```python
from build123d import *

# Parameters (mm, degrees)
SKETCH1_W           = 36.576
SKETCH1_H           = 33.274
BOSS_EXTRUDE1_DEPTH = 1.499997
SKETCH2_W           = 19.05
SKETCH2_H           = 1.5875
SKETCH2_W_2         = 12.7
SKETCH2_W_3         = 9.525
SKETCH2_W_4         = 6.35
SKETCH2_W_5         = 15.875
BOSS_EXTRUDE2_DEPTH = 0.254


with BuildPart() as part:
    # Sketch1 → Boss-Extrude1 (new body)
    with BuildSketch(Plane(origin=(0, 0, 0), x_dir=(1, 0, 0), z_dir=(0, 1, 0))):
        Rectangle(SKETCH1_W, SKETCH1_H)
    extrude(amount=BOSS_EXTRUDE1_DEPTH)

    # Sketch2 → Boss-Extrude2 (add)
    with BuildSketch(Plane(origin=(0, 1.499997, 0), x_dir=(1, 0, 0), z_dir=(0, 1, 0))):
        with Locations((0, 0.66675)):
            Rectangle(SKETCH2_W, SKETCH2_H)
        with Locations((0, -6.31825)):
            Rectangle(SKETCH2_W_2, SKETCH2_H)
        with Locations((0, -9.81075)):
            Rectangle(SKETCH2_W_3, SKETCH2_H)
        with Locations((0, -13.30325)):
            Rectangle(SKETCH2_W_4, SKETCH2_H)
        with Locations((0, -2.82575)):
            Rectangle(SKETCH2_W_5, SKETCH2_H)
    extrude(amount=BOSS_EXTRUDE2_DEPTH)


solid = part.part
```
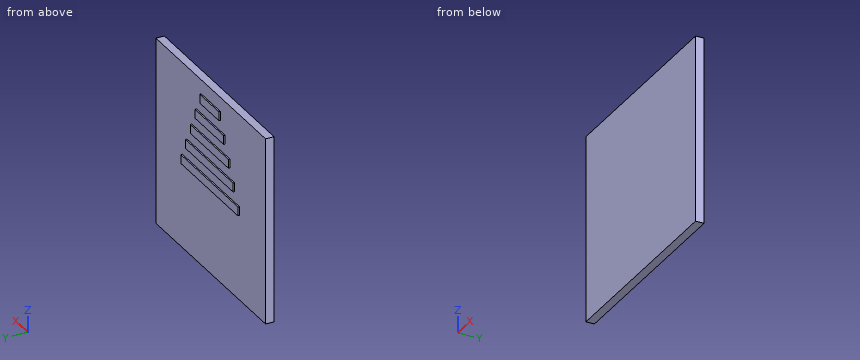
Verification items for the finished model (mm, model axes). Round coordinates to 2 decimals unless told otherwise and drop trailing zeros. Loops run counter-clockwise (first coordinate to the right, second up) from the corner with the lowest first, then second, coordinate; pieces in that order, holes last. Notation, with made-up numbers: (48, 28) -> (55, 28) arc R34 ccw to (55, 58) -> close; hole circle Ø8 at (11.25, 74). An arc over 180 degrees is marked (long way). Answer as a JSON object with one key per item and string values.
Q1. Section check D-D (z = 11.5). Record the boundary of the cut face in (x, y), then the cut area to 3 significant figures.
Data:
{"outline": "(-18.29, 0) -> (18.29, 0) -> (18.29, 1.5) -> (-18.29, 1.5) -> close", "area": "54.9 mm2"}
Q2. Section check A-A (x = -4). Record the boundary of the cut face in (y, z), then the cut area to 3 significant figures.
Data:
{"outline": "(0, -16.64) -> (1.5, -16.64) -> (1.5, -1.46) -> (1.75, -1.46) -> (1.75, 0.13) -> (1.5, 0.13) -> (1.5, 2.03) -> (1.75, 2.03) -> (1.75, 3.62) -> (1.5, 3.62) -> (1.5, 5.52) -> (1.75, 5.52) -> (1.75, 7.11) -> (1.5, 7.11) -> (1.5, 9.02) -> (1.75, 9.02) -> (1.75, 10.6) -> (1.5, 10.6) -> (1.5, 16.64) -> (0, 16.64) -> close", "area": "51.5 mm2"}
Q3. Go/stop test with a flat-tipped pin: P1, Ø1, axis at x = 10.5, z = 9, coming from the +Y side. Record where the tip stops, or that it passes through.
Data:
{"P1": "stops at y = 1.5"}
Q4. Scan line: line 1 (Y direction, x = 6.5, z = 7). Record every from-to range of solid material in increasing order. Write a range as from..to.
Data:
{"line 1": "y = 0..1.5"}
Q5. Section check B-B (z = 3). Record the boundary of the cut face in (x, y), then the cut area to 3 significant figures.
Data:
{"outline": "(-18.29, 0) -> (18.29, 0) -> (18.29, 1.5) -> (7.94, 1.5) -> (7.94, 1.75) -> (-7.94, 1.75) -> (-7.94, 1.5) -> (-18.29, 1.5) -> close", "area": "58.9 mm2"}
Q6. Section check C-C (x = 2.5). Record the boundary of the cut face in (y, z).
Data:
{"outline": "(0, -16.64) -> (1.5, -16.64) -> (1.5, -1.46) -> (1.75, -1.46) -> (1.75, 0.13) -> (1.5, 0.13) -> (1.5, 2.03) -> (1.75, 2.03) -> (1.75, 3.62) -> (1.5, 3.62) -> (1.5, 5.52) -> (1.75, 5.52) -> (1.75, 7.11) -> (1.5, 7.11) -> (1.5, 9.02) -> (1.75, 9.02) -> (1.75, 10.6) -> (1.5, 10.6) -> (1.5, 12.51) -> (1.75, 12.51) -> (1.75, 14.1) -> (1.5, 14.1) -> (1.5, 16.64) -> (0, 16.64) -> close"}
